Can you work these out from the drawing? Everything is in mm from the part's minimum corner. A direction names the side the tool comes from. Give positions to 0.01 mm unless a question says otherwise; leave off trailing zeros. Write each loop counter-clockwise with the first axis right and the second up, starting at its lowest first coordinate (ties: lowest second). Pieces come first, ordered by that corner, then holes. Notation, with made-up numbers: (12.25, -36.75) - (50.25, -36.75) arc R18 ccw to (50.25, -11.75) - close; hole circle Ø10 at (-10, -28.5). An arc over 180 degrees is marked (long way). Use a Markdown table: item, result.
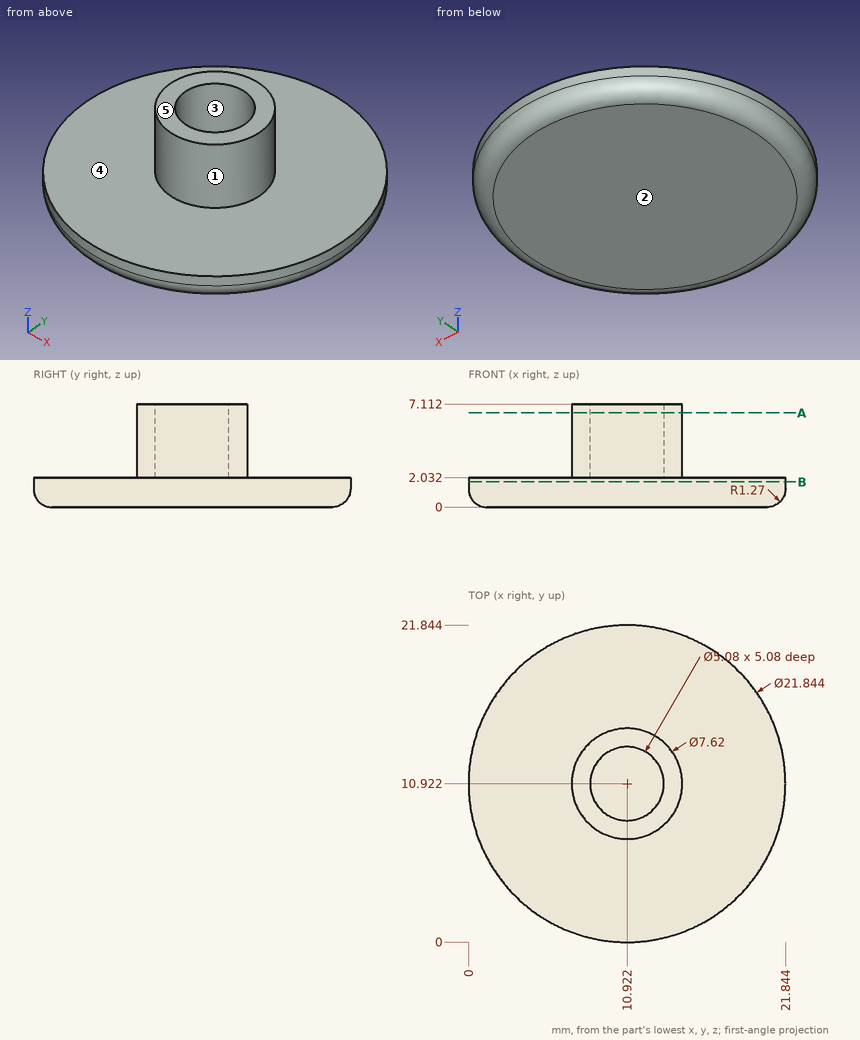
Item 1: If we section it at B-B, the plane z = 1.75: Write out the boundary of the cut face in (x, y), plus the area to 3 significant figures.
Values:
| item | result |
|---|---|
| outline | circle Ø21.84 at (10.92, 10.92) |
| area | 375 mm2 |
Item 2: Will these pins go through, and if not, where does the flat tip stop? pin 1 Ø3 at (y, z) = (2, 4) entering from -X; pin 2 Ø4 at (y, z) = (13.5, 3) entering from -X; pin 3 Ø1.5 at (x, y) = (12, 10.5) entering from +Z.
Values:
| item | result |
|---|---|
| pin 1 | passes through |
| pin 2 | stops at x = 0.03 |
| pin 3 | stops at z = 2.03 |
Item 3: Thinking about a two-plate mould opening in X: for the marked faces 1, 2 and 3, which applies, +X half, -X half, draft (parallel to the pull), parting line (faces both ways), or undercut?
Values:
| item | result |
|---|---|
| face 1 | parting line |
| face 2 | draft |
| face 3 | undercut |
Item 4: For the marked faces 4 and 5, which set-ups out of +Z, -Z, +X, -X, +Y, -Y let a thin tool reach every point of the face, with its end or its side?
Values:
| item | result |
|---|---|
| face 4 | +Z |
| face 5 | +Z, +X, -X, +Y, -Y |
Item 5: I need wall thicknesses on line 1 along X through (y, z) = (10.75, 1.75); line 2 along Z through (x, y) = (11.25, 6); line 3 along Y through (x, z) = (11.75, 2.75). Which ranges of each line are inside material? Lowest first, please. Write a range as [from, to].
Values:
| item | result |
|---|---|
| line 1 | x = [0, 21.84] |
| line 2 | z = [0, 2.03] |
| line 3 | y = [7.2, 8.52], [13.32, 14.64] |
Item 6: If we section it at A-A, the plane z = 6.5: Write out the boundary of the cut face in (x, y), plus the area to 3 significant figures.
Values:
| item | result |
|---|---|
| outline | circle Ø7.62 at (10.92, 10.92); hole circle Ø5.08 at (10.92, 10.92) |
| area | 25.3 mm2 |
